from build123d import *

# Parameters (mm, degrees)
BOSS_EXTRUDE1_DEPTH = 19.05
CUT_EXTRUDE1_DEPTH  = 12.7
FILLET1_R           = 2.54


with BuildPart() as part:
    # Sketch1 → Boss-Extrude1 (new body)
    with BuildSketch(Plane(origin=(0, 0, 0), x_dir=(1, 0, 0), z_dir=(0, 1, 0))):
        with BuildLine():
            Line((57.234735331, 57.711554056), (68.22559355, 65.553540024))
            ThreePointArc((68.22559355, 65.553540024), (0, 94.615), (-68.22559355, 65.553540024))
            Line((-68.22559355, 65.553540024), (-57.234735331, 57.711554056))
            ThreePointArc((-57.234735331, 57.711554056), (0, 81.28), (57.234735331, 57.711554056))
        make_face()
    extrude(amount=BOSS_EXTRUDE1_DEPTH)

    # Sketch3 → Cut-Extrude1 (cut)
    with BuildSketch(Plane.XZ):
        with BuildLine():
            Line((-60.379405736, -59.955278859), (-64.043453365, -62.569579718))
            ThreePointArc((-64.043453365, -62.569579718), (0, -89.535), (64.043453365, -62.569579718))
            Line((64.043453365, -62.569579718), (60.379405736, -59.955278859))
            ThreePointArc((60.379405736, -59.955278859), (0, -85.09), (-60.379405736, -59.955278859))
        make_face()
    extrude(amount=-CUT_EXTRUDE1_DEPTH, mode=Mode.SUBTRACT)

    # Fillet1
    fillet1_edges = [part.edges().sort_by_distance(p)[0] for p in [
        (0, 19.05, -81.28),
        (0, 19.05, -94.615),
    ]]
    fillet(fillet1_edges, radius=FILLET1_R)


solid = part.part
Work out the finished part from the listing and answer in its coordinate system (mm). A direction names the side the tool comes from. Round coordinates to 2 decimals unless told otherwise and drop trailing zeros. Loops run counter-clockwise (first coordinate to the right, second up) from the corner with the lowest first, then second, coordinate; pieces in that order, holes last. Notation, with made-up numbers: (-8.5, 58) - (49.5, 58) arc R19 cw to (49.5, 80) - close; hole circle Ø11 at (37.5, -17). An arc over 180 degrees is marked (long way). Use one line per item in the form item = value. Start each with the question number.
(1) Find section A-A on y = 2.5. Determine the outline of the cut face in (x, z) (3 decimals), and give its area (3 significant figures).
(2) Find section C-C on y = 14.25. Determine the outline of the cut face in (x, z) (3 decimals).
(3) Determine the mould class of faces 3 (the face through (1.07, 8.14, -94.61)), 4 (the face through (-0.889, 8.139, -81.275)), 5 (the face through (0, 0, -82)) for opening direction X: +X half, -X half, draft (parallel to the pull), parting line (faces both ways), or undercut.
(4) Find section B-B on x = 0. Determine the outline of the cut face in (y, z) (3 decimals).
(5) Which of the six approach directions +Z, -Z, +X, -X, +Y, -Y give full straight-line access (tool end or side, diameter ignored) to faces 1 (the face through (0, 12.7, -87)), 2 (the face through (-65.25, 9.39, -63.43))?
(6) Flat-ended cylindrical pins translate along their axes: P1, Ø5, axis at x = 25.5, y = 6.5, coming from the +Z side; P2, Ø1.5, axis at x = 49.5, y = 8.5, coming from the +Z side; P3, Ø1.5, axis at x = 41, z = -85, coming from the +Y side. Find the tip coordinate at first contact, or state that the pin passes through.
(7) Consider line 1 (X direction, y = 10.5, z = -65); line 2 (X direction, y = 5.25, z = -71); line 3 (Z direction, x = -1.5, y = 15.25). Determine where each line is inside the solid, lowest interval first.
Answer list:
q1.outline = (-68.226, -65.554) arc R94.615 ccw to (68.226, -65.554) - (64.043, -62.57) arc R89.535 cw to (-64.043, -62.57) - close; (-60.379, -59.955) arc R85.09 ccw to (60.379, -59.955) - (57.235, -57.712) arc R81.28 cw to (-57.235, -57.712) - close
q1.area = 1,250 mm^2
q2.outline = (-68.226, -65.554) arc R94.615 ccw to (68.226, -65.554) - (57.235, -57.712) arc R81.28 cw to (-57.235, -57.712) - close
q3.face_3 = parting line
q3.face_4 = undercut
q3.face_5 = draft
q4.outline = (0, -94.615) - (16.51, -94.615) arc R2.54 ccw to (19.05, -92.075) - (19.05, -83.82) arc R2.54 ccw to (16.51, -81.28) - (0, -81.28) - (0, -85.09) - (12.7, -85.09) - (12.7, -89.535) - (0, -89.535) - close
q5.face_1 = -Y
q5.face_2 = +Z, -X, +Y, -Y
q6.P1 = -76.3
q6.P2 = -63.89
q6.P3 = 18.52
q7.line_1 = -67.45 to -61.58, -54.91 to -48.8, 48.8 to 54.91, 61.58 to 67.45
q7.line_2 = -62.54 to -54.55, -46.9 to -39.57, 39.57 to 46.9, 54.55 to 62.54
q7.line_3 = -94.6 to -81.27
